The listing builds one solid part. Answer for the finished solid, in the listing's coordinates (mm). Face numbers are marked on the shaded views. A direction names the side the tool comes from. Coordinates: 2 decimals unless noted, no trailing zeros. Loops run counter-clockwise (first coordinate to the right, second up) from the corner with the lowest first, then second, coordinate; pieces in that order, holes last. Notation, with made-up numbers: (1.25, 87.5) - (32.25, 87.5) arc R5 ccw to (32.25, 94.5) - close; hole circle Ø9 at (-3.5, 72.25). An arc over 180 degrees is marked (long way). Put each result on its own line as item: value.
```python
from build123d import *

# Parameters (mm, degrees)
ESQUISSE1_W             = 960
ESQUISSE1_H             = 601.98
BOSS_EXTRU_1_DEPTH      = 285
ESQUISSE4_W             = 947.3
ESQUISSE4_H             = 557.3
ENL_V_MAT_EXTRU_7_DEPTH = 595.63
ESQUISSE5_W             = 557.3
ESQUISSE5_H             = 40
ENL_V_MAT_EXTRU_8_DEPTH = 1046.667241574
ESQUISSE6_W             = 304.8
ESQUISSE6_H             = 254
ENL_V_MAT_EXTRU_9_DEPTH = 25.4


with BuildPart() as part:
    # Esquisse1 → Boss.-Extru.1 (new, symmetric)
    with BuildSketch(Plane.XY):
        Rectangle(ESQUISSE1_W, ESQUISSE1_H)
    extrude(amount=BOSS_EXTRU_1_DEPTH, both=True)

    # Esquisse4 → Enlèv. mat.-Extru.7 (cut)
    with BuildSketch(Plane.XZ.offset(300.99)):
        Rectangle(ESQUISSE4_W, ESQUISSE4_H)
    extrude(amount=-ENL_V_MAT_EXTRU_7_DEPTH, mode=Mode.SUBTRACT)

    # Esquisse5 → Enlèv. mat.-Extru.8 (cut, through all)
    with BuildSketch(Plane(origin=(480, 0, 0), x_dir=(0, 0, -1), z_dir=(1, 0, 0))):
        with Locations((0, -280.99)):
            Rectangle(ESQUISSE5_W, ESQUISSE5_H)
    extrude(amount=-ENL_V_MAT_EXTRU_8_DEPTH, mode=Mode.SUBTRACT)

    # Esquisse6 → Enlèv. mat.-Extru.9 (cut)
    with BuildSketch(Plane.XY.offset(285)):
        with Locations((0, -97.79)):
            Rectangle(ESQUISSE6_W, ESQUISSE6_H)
    extrude(amount=-ENL_V_MAT_EXTRU_9_DEPTH, mode=Mode.SUBTRACT)


solid = part.part
```
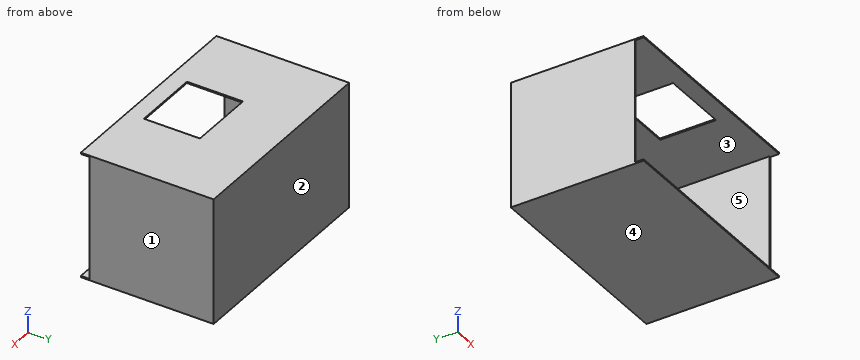
1) Straight lines are drawn through the part: L1, parallel to Z at x = -428, y = -248; L2, parallel to X at y = 175.5, z = -217; L3, parallel to Y at x = -362, z = 88. For each, find the intervals that lie inside material, in ascending order. Write a range as [from, to].
Found:
L1: z = [-285, -278.65], [278.65, 285]
L2: x = [-480, -473.65], [473.65, 480]
L3: y = [294.64, 300.99]
2) The part is cut by section B-B (y = -186). Give the vertices of the cut face in (x, z).
Found:
outline: (-480, -285) - (480, -285) - (480, 285) - (152.4, 285) - (152.4, 278.65) - (473.65, 278.65) - (473.65, -278.65) - (-473.65, -278.65) - (-473.65, 278.65) - (-152.4, 278.65) - (-152.4, 285) - (-480, 285) - close
3) Each of these flat-tipped pins is pushed along its axis until it touches: pin 1 (1.9 mm diameter, centred on x = 475.5, z = -108.5, fed in from -Y); pin 2 (8 mm diameter, centred on x = -141, y = -199, fed in from +Z); pin 3 (3 mm diameter, centred on x = -154.5, z = -37.5, fed in from -Y). Where does it stop, or does it pass through?
Found:
pin 1: stops at y = -260.99
pin 2: stops at z = -278.65
pin 3: stops at y = 294.64
4) The part is cut by section C-C (z = 179). Give the vertices of the cut face in (x, y), and give its area (3 significant figures).
Found:
outline: (-480, -260.99) - (-473.65, -260.99) - (-473.65, 294.64) - (473.65, 294.64) - (473.65, -260.99) - (480, -260.99) - (480, 300.99) - (-480, 300.99) - close
area: 13,200 mm^2
5) The part is cut by section D-D (y = 127.5). Give the vertices of the cut face in (x, z), and give its area (3 significant figures).
Found:
outline: (-480, -285) - (480, -285) - (480, 285) - (-480, 285) - close; hole (-473.65, -278.65) - (473.65, -278.65) - (473.65, 278.65) - (-473.65, 278.65) - close
area: 19,300 mm^2
6) For the marked faces 4 and 5, determine the directions among +Z, -Z, +X, -X, +Y, -Y from which every point of the face is accessible in a straight line to the end or side of a thin tool.
Found:
face 4: -Z, +X, -X, +Y, -Y
face 5: -Y
7) For a pull along X with two mould halves and no side action, classify the marked faces 1, 2 and 3 as pulls with the +X half, pulls with the -X half, needs draft (parallel to the pull), parting line crosses it, or undercut.
Found:
face 1: pulls with the +X half
face 2: needs draft
face 3: undercut
8) The part is cut by section A-A (x = 141). Give the vertices of the cut face in (y, z).
Found:
outline: (-300.99, -285) - (300.99, -285) - (300.99, 285) - (29.21, 285) - (29.21, 278.65) - (294.64, 278.65) - (294.64, -278.65) - (-300.99, -278.65) - close; (-300.99, 278.65) - (-224.79, 278.65) - (-224.79, 285) - (-300.99, 285) - close
